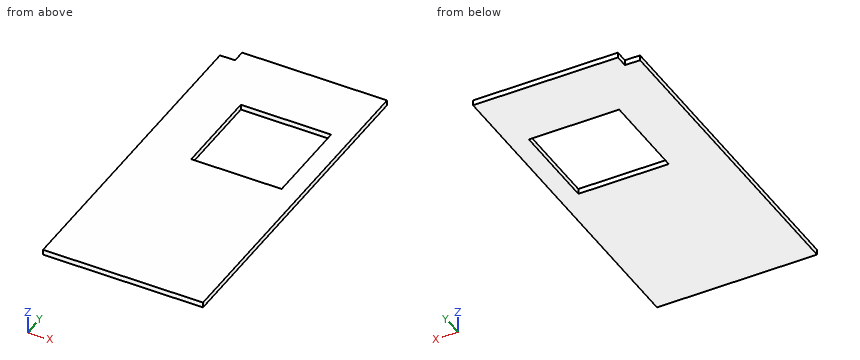
from build123d import *

# Parameters (mm, degrees)
SKETCH1_W           = 1146.302
SKETCH1_H           = 2405.888
SKETCH1_W_2         = 647.7
SKETCH1_H_2         = 647.7
BOSS_EXTRUDE1_DEPTH = 38.1
SKETCH2_W           = 108.204
SKETCH2_H           = 91.948
CUT_EXTRUDE1_DEPTH  = 38.1


with BuildPart() as part:
    # Sketch1 → Boss-Extrude1 (new body)
    with BuildSketch(Plane.XY):
        Rectangle(SKETCH1_W, SKETCH1_H)
        with Locations((113.157, 397.764)):
            Rectangle(SKETCH1_W_2, SKETCH1_H_2, mode=Mode.SUBTRACT)
    extrude(amount=BOSS_EXTRUDE1_DEPTH)

    # Sketch2 → Cut-Extrude1 (cut)
    with BuildSketch(Plane.XY.offset(38.1)):
        with Locations((-519.049, 1156.97)):
            Rectangle(SKETCH2_W, SKETCH2_H)
    extrude(amount=-CUT_EXTRUDE1_DEPTH, mode=Mode.SUBTRACT)


solid = part.part
Design review of the part built by this model. Coordinates are the model's own, in mm. Coordinates: 2 decimals unless noted, no trailing zeros. Order: outer loops, then holes, each group sorted by start corner. A loop starts at its lowest first (then second) coordinate and runs counter-clockwise, first axis right, second up. Notation, with made-up numbers: (-21, 79) -> (-14, 79) arc R21 cw to (-14, 88) -> close; hole circle Ø8 at (4.5, 69.25). An arc over 180 degrees is marked (long way). Use one line per item in the form item = value. Start each with the question number.
(1) Add section C-C on z = 9.5. State the section outline as (x, y) points, plus the area to 3 significant figures.
(2) Add section B-B on y = 131. State the section outline as (x, z) points.
(3) For probe 1 along X at (y, z) = (265, 33.5); probe 2 along Y at (x, z) = (203.5, 25); probe 3 along Y at (x, z) = (-482, 31), list the stretches that pass through material, from the lowest coordinate up.
(4) Add section A-A on x = 77. State the section outline as (y, z) points, plus the area to 3 significant figures.
(5) Insertion check: pin 1 (4 mm diameter, centred on x = -339.5, y = 492.5, fed in from -Z). The pin has a flat end and moves straight along its axis. Give the tip position at first contact, or say it passes through.
Answer block:
q1.outline = (-573.15, -1202.94) -> (573.15, -1202.94) -> (573.15, 1202.94) -> (-464.95, 1202.94) -> (-464.95, 1111) -> (-573.15, 1111) -> close; hole (-210.69, 73.91) -> (437.01, 73.91) -> (437.01, 721.61) -> (-210.69, 721.61) -> close
q1.area = 2,330,000 mm²
q2.outline = (-573.15, 0) -> (-210.69, 0) -> (-210.69, 38.1) -> (-573.15, 38.1) -> close; (437.01, 0) -> (573.15, 0) -> (573.15, 38.1) -> (437.01, 38.1) -> close
q3.probe_1 = -573.15 to -210.69, 437.01 to 573.15
q3.probe_2 = -1202.94 to 73.91, 721.61 to 1202.94
q3.probe_3 = -1202.94 to 1111
q4.outline = (-1202.94, 0) -> (73.91, 0) -> (73.91, 38.1) -> (-1202.94, 38.1) -> close; (721.61, 0) -> (1202.94, 0) -> (1202.94, 38.1) -> (721.61, 38.1) -> close
q4.area = 67,000 mm²
q5.pin_1 = 0
